Design review of the part built by this model. Coordinates are the model's own, in mm. A direction names the side the tool comes from. Give positions to 0.01 mm unless a question says otherwise; leave off trailing zeros. Order: outer loops, then holes, each group sorted by start corner. A loop starts at its lowest first (then second) coordinate and runs counter-clockwise, first axis right, second up.
```python
from build123d import *

# Parameters (mm, degrees)
RESSALTO_EXTRUS_O1_DEPTH = 10
ESBO_O2_R                = 2.5
CORTE_EXTRUS_O1_DEPTH    = 218.763914705
RESSALTO_EXTRUS_O2_DEPTH = 30
ESBO_O5_R                = 2.5
CORTE_EXTRUS_O2_DEPTH    = 5
ESBO_O6_R                = 2.5
CORTE_EXTRUS_O3_DEPTH    = 5
CORTE_EXTRUS_O4_DEPTH    = 10


with BuildPart() as part:
    # Esboço1 → Ressalto-extrusão1 (new body)
    with BuildSketch(Plane(origin=(0, 0, 0), x_dir=(1, 0, 0), z_dir=(0, 1, 0))):
        with BuildLine():
            Line((-88.275862069, -57.715517241), (91.724137931, -57.715517241))
            ThreePointArc((91.724137931, -57.715517241), (98.795205743, -54.786585053), (101.724137931, -47.715517241))
            Line((101.724137931, -47.715517241), (101.724137931, 182.284482759))
            ThreePointArc((101.724137931, 182.284482759), (98.795205743, 189.35555057), (91.724137931, 192.284482759))
            Line((91.724137931, 192.284482759), (-88.275862069, 192.284482759))
            ThreePointArc((-88.275862069, 192.284482759), (-95.346929881, 189.35555057), (-98.275862069, 182.284482759))
            Line((-98.275862069, 182.284482759), (-98.275862069, -47.715517241))
            ThreePointArc((-98.275862069, -47.715517241), (-95.346929881, -54.786585053), (-88.275862069, -57.715517241))
        make_face()
    extrude(amount=RESSALTO_EXTRUS_O1_DEPTH)

    # Esboço2 → Corte-extrusão1 (cut, through all)
    with BuildSketch(Plane(origin=(0, 10, 0), x_dir=(1, 0, 0), z_dir=(0, 1, 0))):
        with Locations(Location((-83.275862069, 102.284482759, 0), (0, 0, 270))):
            Circle(ESBO_O2_R)
        with Locations(Location((86.724137931, 177.284482759, 0), (0, 0, 90))):
            Circle(ESBO_O2_R)
        with Locations(Location((86.724137931, -42.715517241, 0), (0, 0, 270))):
            Circle(ESBO_O2_R)
        with Locations(Location((-83.275862069, 32.284482759, 0), (0, 0, 90))):
            Circle(ESBO_O2_R)
        with BuildLine():
            Line((31.724137931, 107.284482759), (-28.275862069, 107.284482759))
            ThreePointArc((-28.275862069, 107.284482759), (-35.346929881, 104.35555057), (-38.275862069, 97.284482759))
            Line((-38.275862069, 97.284482759), (-38.275862069, 37.284482759))
            ThreePointArc((-38.275862069, 37.284482759), (-35.346929881, 30.213414947), (-28.275862069, 27.284482759))
            Line((-28.275862069, 27.284482759), (31.724137931, 27.284482759))
            ThreePointArc((31.724137931, 27.284482759), (38.795205743, 30.213414947), (41.724137931, 37.284482759))
            Line((41.724137931, 37.284482759), (41.724137931, 97.284482759))
            ThreePointArc((41.724137931, 97.284482759), (38.795205743, 104.35555057), (31.724137931, 107.284482759))
        make_face()
    extrude(amount=-CORTE_EXTRUS_O1_DEPTH, mode=Mode.SUBTRACT)

    # Esboço4 → Ressalto-extrusão2 (add)
    with BuildSketch(Plane(origin=(0, 10, 0), x_dir=(1, 0, 0), z_dir=(0, 1, 0))):
        Polygon((58.224137931, 9.784482759), (-38.275862069, 9.784482759), (-38.275862069, 4.784482759), (63.224137931, 4.784482759), align=None)
        Polygon((58.224137931, 124.784482759), (-38.275862069, 124.784482759), (-38.275862069, 129.784482759), (63.224137931, 129.784482759), align=None)
    extrude(amount=RESSALTO_EXTRUS_O2_DEPTH)

    # Esboço5 → Corte-extrusão2 (cut)
    with BuildSketch(Plane.XY.offset(-4.784482759)):
        with Locations((-30.275862069, 20.836178243)):
            Circle(ESBO_O5_R)
        with Locations((28.724137931, 19.5)):
            Circle(ESBO_O5_R)
    extrude(amount=-CORTE_EXTRUS_O2_DEPTH, mode=Mode.SUBTRACT)

    # Esboço6 → Corte-extrusão3 (cut)
    with BuildSketch(Plane(origin=(0, 0, -129.784482759), x_dir=(-1, 0, 0), z_dir=(0, 0, -1))):
        with Locations((-31.724137931, 19.5)):
            Circle(ESBO_O6_R)
        with Locations((30.275862069, 17.5)):
            Circle(ESBO_O6_R)
    extrude(amount=-CORTE_EXTRUS_O3_DEPTH, mode=Mode.SUBTRACT)

    # Esboço7 → Corte-extrusão4 (cut)
    with BuildSketch(Plane(origin=(0, 10, 0), x_dir=(1, 0, 0), z_dir=(0, 1, 0))):
        with BuildLine():
            Line((76.724137931, 117.284482759), (71.724137931, 117.284482759))
            ThreePointArc((71.724137931, 117.284482759), (64.653070119, 114.35555057), (61.724137931, 107.284482759))
            Line((61.724137931, 107.284482759), (61.724137931, 27.284482759))
            ThreePointArc((61.724137931, 27.284482759), (64.653070119, 20.213414947), (71.724137931, 17.284482759))
            Line((71.724137931, 17.284482759), (76.724137931, 17.284482759))
            ThreePointArc((76.724137931, 17.284482759), (83.795205743, 20.213414947), (86.724137931, 27.284482759))
            Line((86.724137931, 27.284482759), (86.724137931, 107.284482759))
            ThreePointArc((86.724137931, 107.284482759), (83.795205743, 114.35555057), (76.724137931, 117.284482759))
        make_face()
        with BuildLine():
            Line((-58.289420658, 116.784482759), (-63.289420658, 116.784482759))
            ThreePointArc((-63.289420658, 116.784482759), (-70.36048847, 113.85555057), (-73.289420658, 106.784482759))
            Line((-73.289420658, 106.784482759), (-73.289420658, 26.784482759))
            ThreePointArc((-73.289420658, 26.784482759), (-70.36048847, 19.713414947), (-63.289420658, 16.784482759))
            Line((-63.289420658, 16.784482759), (-58.289420658, 16.784482759))
            ThreePointArc((-58.289420658, 16.784482759), (-51.218352846, 19.713414947), (-48.289420658, 26.784482759))
            Line((-48.289420658, 26.784482759), (-48.289420658, 106.784482759))
            ThreePointArc((-48.289420658, 106.784482759), (-51.218352846, 113.85555057), (-58.289420658, 116.784482759))
        make_face()
    extrude(amount=-CORTE_EXTRUS_O4_DEPTH, mode=Mode.SUBTRACT)


solid = part.part
```
1. For line 1 along X through (y, z) = (2.5, -36.5); line 2 along Z through (x, y) = (-30, 31.5); line 3 along Y through (x, z) = (-52.5, -7), list the stretches that pass through material, from the lowest coordinate up.
Recorded:
line 1: x = -98.28 to -73.29, -48.29 to -38.25, 41.69 to 61.72, 86.72 to 101.72
line 2: z = -129.78 to -124.78, -9.78 to -4.78
line 3: y = 0 to 10
2. Machinability: for faces 5 (the face through (45, 0, -69)), 6 (the face through (60.76, 24.79, -127.32)), 7 (the face through (86.724, 5, -67)), 8 (the face through (-32.773, 20.946, -7.249)), 9 (the face through (-38.276, 25, -7)), which of the approach directions +Z, -Z, +X, -X, +Y, -Y give a long, thin tool a straight path to every point of the face, cutting with its end or side? Answer none if there is none.
Recorded:
face 5: +Z, -Z, +X, -X, -Y
face 6: +X, +Y
face 7: +Y, -Y
face 8: +Z
face 9: +Z, -Z, -X, +Y
3. For pin 1 (3 mm diameter, centred on x = 55.5, z = -23, fed in from +Y); pin 2 (4 mm diameter, centred on y = 27, z = -127, fed in from -X); pin 3 (9 mm diameter, centred on x = 0.5, y = 26.5, fed in from +Z); pin 4 (1 mm diameter, centred on x = -72, z = -34.5, fed in from -Y), all flat-tipped, find the tip position at first contact; note any pin that passes through.
Recorded:
pin 1: stops at y = 10
pin 2: stops at x = -38.28
pin 3: stops at z = -4.78
pin 4: passes through
4. Take a section at C-C (x = -42). State the section outline as (y, z) points.
Recorded:
outline: (0, -192.28) - (10, -192.28) - (10, 57.72) - (0, 57.72) - close
5. Take a section at D-D (z = 3). State the section outline as (x, y) points.
Recorded:
outline: (-98.28, 0) - (101.72, 0) - (101.72, 10) - (-98.28, 10) - close
6. Draft analysis for pull direction X (two halves, no side actions). For faces 1 (the face through (74, 5, -17.284)), 2 (the face through (-51.297, 5.07, -19.636)), 3 (the face through (-95.3, 4.9, -189.4)), 4 (the face through (0, 5, 57.716)), state which applies: pulls with the +X half, pulls with the -X half, needs draft (parallel to the pull), parting line crosses it, or undercut.
Recorded:
face 1: undercut
face 2: undercut
face 3: pulls with the -X half
face 4: needs draft
7. Take a section at A-A (y = 26.5). State the section outline as (x, z) points.
Recorded:
outline: (-38.28, -129.78) - (63.22, -129.78) - (58.22, -124.78) - (-38.28, -124.78) - close; (-38.28, -9.78) - (58.22, -9.78) - (63.22, -4.78) - (-38.28, -4.78) - close
8. Take a section at B-B (x = 11). State the section outline as (y, z) points, then the cut area to 3 significant figures.
Recorded:
outline: (0, -192.28) - (10, -192.28) - (10, -129.78) - (40, -129.78) - (40, -124.78) - (10, -124.78) - (10, -107.28) - (0, -107.28) - close; (0, -27.28) - (10, -27.28) - (10, -9.78) - (40, -9.78) - (40, -4.78) - (10, -4.78) - (10, 57.72) - (0, 57.72) - close
area: 2,000 mm2
